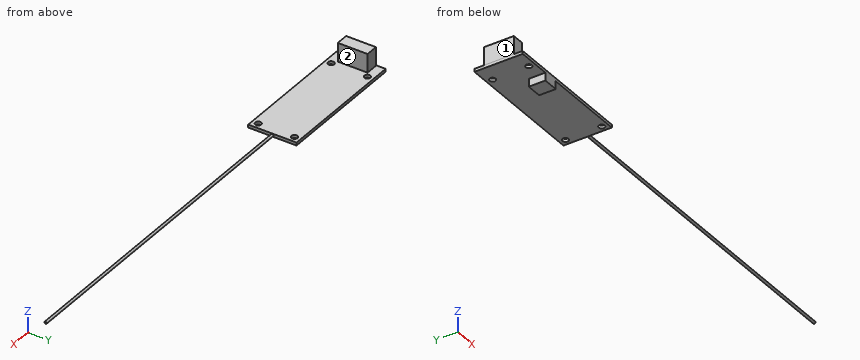
```python
from build123d import *

# Parameters (mm, degrees)
SKETCH1_W                             = 69.85
SKETCH1_H                             = 25.4
EXTRUDE1_DEPTH                        = 1.5748
F_1_8_0_125_DIAMETER_HOLE1_AT_2_COUNT = 2
F_1_8_0_125_DIAMETER_HOLE1_AT_2_PITCH = 57.13222
SKETCH4_R                             = 0.635
BOSS_EXTRUDE1_DEPTH                   = 177.8
SKETCH5_W                             = 8.128
SKETCH5_H                             = 8.7376
USB_CONNECTOR_DEPTH                   = 4.1402
SKETCH8_W                             = 6.5278
SKETCH8_H                             = 15.6718
BOSS_EXTRUDE3_DEPTH                   = 9.8298


with BuildPart() as part:
    # Sketch1 → Extrude1 (new body)
    with BuildSketch(Plane.XY):
        Rectangle(SKETCH1_W, SKETCH1_H)
    extrude(amount=EXTRUDE1_DEPTH)

    # Sketch3 → 1/8 (0.125) Diameter Hole1 (revolve, cut)
    with BuildSketch(Plane(origin=(-25.38222, 9.525, 1.5748), x_dir=(0, -1, 0), z_dir=(1, 0, 0))):
        Polygon((0, 0), (0, 16.955866233), (1.5875, 16.002), (1.5875, 0), align=None)
    f_1_8_0_125_diameter_hole1 = revolve(axis=Axis((-25.38222, 9.525, 7.9248), (0, 0, -1)), mode=Mode.SUBTRACT)

    # 1/8 (0.125) Diameter Hole1 at 2: 1/8 (0.125) Diameter Hole1 ×2
    with Locations(*[(i * F_1_8_0_125_DIAMETER_HOLE1_AT_2_PITCH, 0, 0) for i in range(1, F_1_8_0_125_DIAMETER_HOLE1_AT_2_COUNT)]):
        add(f_1_8_0_125_diameter_hole1, mode=Mode.SUBTRACT)

    # Mirror1: 1/8 (0.125) Diameter Hole1 across plane
    add(f_1_8_0_125_diameter_hole1.mirror(Plane.ZX), mode=Mode.SUBTRACT)

    # Mirror1 copy 1 sketch → Mirror1 copy 1 (revolve, cut)
    with BuildSketch(Plane(origin=(31.75, -9.525, 1.5748), x_dir=(0, 1, 0), z_dir=(1, 0, 0))):
        Polygon((0, 0), (0, -16.955866233), (1.5875, -16.002), (1.5875, 0), align=None)
    revolve(axis=Axis((31.75, -9.525, 7.9248), (0, 0, 1)), mode=Mode.SUBTRACT)

    # Sketch4 → Boss-Extrude1 (add)
    with BuildSketch(Plane(origin=(34.925, 0, 0), x_dir=(0, 0, -1), z_dir=(1, 0, 0))):
        with Locations(Location((-0.772028936, 0, 0), (0, 0, 180))):
            Circle(SKETCH4_R)
    extrude(amount=BOSS_EXTRUDE1_DEPTH)

    # Sketch5 → USB Connector (add)
    with BuildSketch(Plane(origin=(0, 0, 0), x_dir=(-1, 0, 0), z_dir=(0, 0, -1))):
        with Locations((13.072066229, -8.3312)):
            Rectangle(SKETCH5_W, SKETCH5_H)
    extrude(amount=USB_CONNECTOR_DEPTH)

    # Sketch8 → Boss-Extrude3 (add)
    with BuildSketch(Plane.XY.offset(1.5748)):
        with Locations((-31.2801, 0)):
            Rectangle(SKETCH8_W, SKETCH8_H)
    extrude(amount=BOSS_EXTRUDE3_DEPTH)


solid = part.part
```
Geometry check sheet. Reference: the model listing, model coordinates, mm. Face numbers are marked on the shaded views. A direction names the side the tool comes from. Coordinates: 2 decimals unless noted, no trailing zeros. Order: outer loops, then holes, each group sorted by start corner. A loop starts at its lowest first (then second) coordinate and runs counter-clockwise, first axis right, second up.
Q1. Sectioned sample at A-A on y = 4. Record the cut outline in (x, z) (3 decimals), and give its area (3 significant figures).
Reply:
outline: (-34.925, 0) - (34.925, 0) - (34.925, 1.575) - (-28.016, 1.575) - (-28.016, 11.405) - (-34.544, 11.405) - (-34.544, 1.575) - (-34.925, 1.575) - close
area: 174 mm2
Q2. Sectioned sample at D-D on x = -7. Record the cut outline in (y, z), and give its area (3 significant figures).
Reply:
outline: (-12.7, 0) - (12.7, 0) - (12.7, 1.57) - (-12.7, 1.57) - close
area: 40.0 mm2
Q3. Thickness scan on probe 1 along Y at (x, z) = (31.75, 0.3); probe 2 along X at (y, z) = (8.5, 1.25) (3 decimals); probe 3 along X at (y, z) = (-7.25, 9.5). Record the ranges inside material, lowest first.
Reply:
probe 1: y = -12.7 to -11.11, -7.94 to 7.94, 11.11 to 12.7
probe 2: x = -34.925 to -26.594, -24.17 to 30.538, 32.962 to 34.925
probe 3: x = -34.54 to -28.02
Q4. Sectioned sample at B-B on z = -2. Record the cut outline in (x, y).
Reply:
outline: (-17.14, -12.7) - (-9.01, -12.7) - (-9.01, -3.96) - (-17.14, -3.96) - close
Q5. Tool access check on the marked faces 1 and 2. Record the directions out of +Z, -Z, +X, -X, +Y, -Y that give a thin tool (end or side, any length) a straight path to the whole face; none if there is none.
Reply:
face 1: +Z, -X, +Y, -Y
face 2: +Z, +X, +Y, -Y
Q6. Sectioned sample at C-C on x = 192.5. Record the cut outline in (y, z) (3 decimals), and give its area (3 significant figures).
Reply:
outline: circle Ø1.27 at (0, 0.772)
area: 1.27 mm2
Q7. Depth check by flat-ended pin: pin 1 Ø12.5 at (x, y) = (5, 1) entering from +Z; pin 2 Ø8 at (y, z) = (1, 8.5) entering from -X; pin 3 Ø1.2 at (y, z) = (-10, -1.5) entering from +X. Enter the tip coordinate at first touch or a pass-through.
Reply:
pin 1: stops at z = 1.57
pin 2: stops at x = -34.54
pin 3: stops at x = -9.01
